Geometry: final body of the model. Coordinates: model frame, mm. Face numbers are marked on the shaded views. A direction names the side the tool comes from. Give positions to 0.01 mm unless a question says otherwise; leave off trailing zeros. Write each loop counter-clockwise with the first axis right and the second up, starting at its lowest first coordinate (ties: lowest second). Pieces come first, ordered by that corner, then holes.
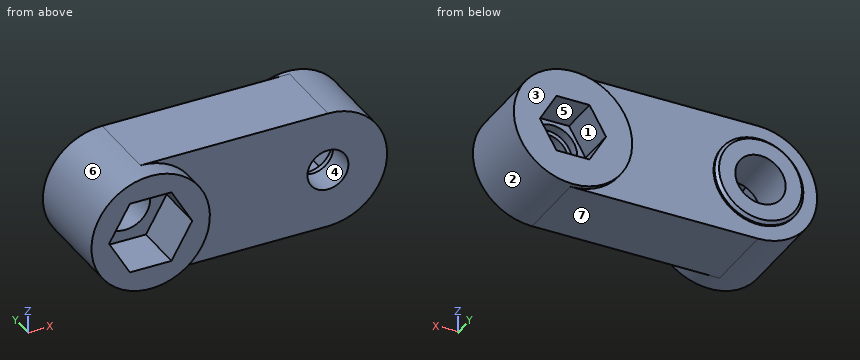
from build123d import *

# Parameters (mm, degrees)
EXTRUDE_1_DEPTH     = 10
CUT_EXTRUDE_1_DEPTH = 5
SKETCH_6_R          = 27.317981471
SKETCH_6_R_2        = 6
CUT_EXTRUDE_2_DEPTH = 2
CUT_EXTRUDE_3_DEPTH = 4
CUT_EXTRUDE_START   = -0.5
SKETCH_8_W          = 36.274656105
SKETCH_8_H          = 16.774008436
SKETCH_8_R          = 6
CUT_EXTRUDE_4_DEPTH = 0.5
SKETCH_9_R          = 6
SKETCH_9_R_2        = 4.5
CUT_EXTRUDE_5_DEPTH = 0.5
CHAMFER_1_SIZE      = 0.3


with BuildPart() as part:
    # 草图1 → 凸台-拉伸1 (new body)
    with BuildSketch(Plane(origin=(0, 0, 0), x_dir=(1, 0, 0), z_dir=(0, 1, 0))):
        with BuildLine():
            Line((0, 6), (19, 6))
            ThreePointArc((19, 6), (25, 0), (19, -6))
            Line((19, -6), (0, -6))
            ThreePointArc((0, -6), (-6, 0), (0, 6))
        make_face()
    extrude(amount=EXTRUDE_1_DEPTH)

    # 草图3 → 切除-旋转2 (revolve, cut)
    with BuildSketch(Plane.XY, mode=Mode.PRIVATE) as cut_revolve_2_sk:
        Polygon((0, 10), (-2.55, 10), (-2.55, 5), (-2.1, 5), (-2.1, 2), (-2.55, 2), (-2.55, 0), (0, 0), align=None)
    revolve(cut_revolve_2_sk.sketch.rotate(Axis((0, 10, 0), (0, -1, 0)), 270), axis=Axis((0, 10, 0), (0, -1, 0)), mode=Mode.SUBTRACT)

    # 草图4 → 切除-旋转3 (revolve, cut)
    with BuildSketch(Plane.XY, mode=Mode.PRIVATE) as cut_revolve_3_sk:
        Polygon((19, 10), (16.5, 10), (16.5, 5), (16.925, 5), (16.925, 0), (19, 0), align=None)
    revolve(cut_revolve_3_sk.sketch.rotate(Axis((19, 10, 0), (0, -1, 0)), 270), axis=Axis((19, 10, 0), (0, -1, 0)), mode=Mode.SUBTRACT)

    # 草图5 → 切除-拉伸1 (cut)
    with BuildSketch(Plane.XZ):
        Polygon((-4.214656965, 0), (-2.107328483, -3.65), (2.107328483, -3.65), (4.214656965, 0), (2.107328483, 3.65), (-2.107328483, 3.65), align=None)
    extrude(amount=-CUT_EXTRUDE_1_DEPTH, mode=Mode.SUBTRACT)

    # 草图6 → 切除-拉伸2 (cut)
    with BuildSketch(Plane.XZ):
        Circle(SKETCH_6_R)
        with Locations(Location((0, 0, 0), (0, 0, 90))):
            Circle(SKETCH_6_R_2, mode=Mode.SUBTRACT)
    extrude(amount=-CUT_EXTRUDE_2_DEPTH, mode=Mode.SUBTRACT)

    # 草图7 → 切除-拉伸3 (cut)
    with BuildSketch(Plane(origin=(0, 10, 0), x_dir=(1, 0, 0), z_dir=(0, 1, 0))):
        Polygon((17.325684219, 2.9), (15.651368439, 0), (17.325684219, -2.9), (20.674315781, -2.9), (22.348631561, 0), (20.674315781, 2.9), align=None)
    extrude(amount=-CUT_EXTRUDE_3_DEPTH, mode=Mode.SUBTRACT)

    # 草图8 → 切除-拉伸4 (cut)
    with BuildSketch(Plane(origin=(0, 10, 0), x_dir=(1, 0, 0), z_dir=(0, 1, 0)).offset(CUT_EXTRUDE_START)):
        with Locations((9.154855794, 0.069028841)):
            Rectangle(SKETCH_8_W, SKETCH_8_H)
        with Locations(Location((0, 0, 0), (0, 0, 270))):
            Circle(SKETCH_8_R, mode=Mode.SUBTRACT)
        with Locations(Location((19, 0, 0), (0, 0, 270))):
            Circle(SKETCH_8_R, mode=Mode.SUBTRACT)
    extrude(amount=CUT_EXTRUDE_4_DEPTH, mode=Mode.SUBTRACT)

    # 草图9 → 切除-拉伸5 (cut)
    with BuildSketch(Plane(origin=(0, 10, 0), x_dir=(1, 0, 0), z_dir=(0, 1, 0)).offset(CUT_EXTRUDE_START)):
        with Locations(Location((0, 0, 0), (0, 0, 270))):
            Circle(SKETCH_9_R)
        with Locations(Location((0, 0, 0), (0, 0, 270))):
            Circle(SKETCH_9_R_2, mode=Mode.SUBTRACT)
    extrude(amount=CUT_EXTRUDE_5_DEPTH, mode=Mode.SUBTRACT)

    # 倒角1
    chamfer_1_edges = [part.edges().sort_by_distance(p)[0] for p in [
        (0, 10, -4.5),
    ]]
    chamfer(chamfer_1_edges, length=CHAMFER_1_SIZE)


solid = part.part
Q1. Pin query (flat end, axial travel): P1, Ø4, axis at x = 0, z = 0, coming from the +Y side; P2, Ø2, axis at x = 21, y = 7.5, coming from the -Z side. Return the tip coordinate at first contact, or that it passes through.
Filled sheet:
P1: passes through
P2: stops at z = -5.92
Q2. Pull-direction query (Z, two-part tool) for the marked faces 1, 2, 3 and 4; classes: released by +Z, released by -Z, zero draft, split by the parting line, or undercut.
Filled sheet:
face 1: undercut
face 2: split by the parting line
face 3: zero draft
face 4: undercut
Q3. Access query for the marked faces 5, 6 and 7. Directions: +Z, -Z, +X, -X, +Y, -Y. A direction counts if a zero-diameter tool reaches every point of the face in a straight line with its end or side. Return the directions, or none.
Filled sheet:
face 5: +Y
face 6: -Y
face 7: -Z, +X, -X, +Y, -Y
Q4. Ray query, line 1 along Z through (x, y) = (19, 2.9) (3 decimals); line 2 along Z through (x, y) = (0.5, 8.5); line 3 along Y through (x, z) = (22, -2.75). Return the intervals inside material, ascending.
Filled sheet:
line 1: z = -6 to -2.075, 2.075 to 6
line 2: z = -6 to -2.5, 2.5 to 6
line 3: y = 2 to 10
Q5. Section A-A on y = 3.25. Output: boundary loops of the cut face in (x, z) (3 decimals).
Filled sheet:
outline: (0, -6) - (19, -6) arc R6 ccw to (19, 6) - (0, 6) arc R6 ccw to start; hole (-4.215, 0) - (-2.107, -3.65) - (2.107, -3.65) - (4.215, 0) - (2.107, 3.65) - (-2.107, 3.65) - close; hole circle Ø4.15 at (19, 0)
Q6. Section C-C on z = 0.75. Count the separate pieces of the cut face and the enclosed holes in it, plus the area to 3 significant figures.
Filled sheet:
separate pieces: 3
enclosed holes: 0
area: 164 mm2
